Check sheet for the modelled part. Datum: model origin and axes. Units: mm. Face numbers are marked on the shaded views. A direction names the side the tool comes from. Round coordinates to 2 decimals unless told otherwise and drop trailing zeros. Loops run counter-clockwise (first coordinate to the right, second up) from the corner with the lowest first, then second, coordinate; pieces in that order, holes last. Notation, with made-up numbers: M 52.5,68.25 L 102.5,68.25 A19 cw 102.5,81.25 Z; hole C 78.5,59.25 d6. An arc over 180 degrees is marked long. One line per question, with ' | ' between items. Start each with the question number.
(1) Draft check along X on the marked faces 3, 4 and 5. Enter one of: +X half, -X half, draft (parallel to the pull), parting line (faces both ways), or undercut.
(2) Thickness scan on probe 1 along Z at (x, y) = (-44, -1); probe 2 along X at (y, z) = (-3.5, 36); probe 3 along Y at (x, z) = (-59, 32) (3 decimals). Record the ranges inside material, lowest first. Write a range as [from, to].
(3) Section check B-B (y = -4.25). Record the boundary of the cut face in (x, z) (3 decimals).
(4) Go/stop test with flat-tipped pins: P1, Ø2, axis at y = -2.5, z = 44.5, coming from the -X side; P2, Ø1, axis at x = -41.5, y = -4.5, coming from the -Z side; P3, Ø1.5, axis at y = -4.5, z = 38, coming from the +X side. Record where each tip stops, or that it passes through.
(5) Tool access check on the marked faces 1 and 2. Record the directions out of +Z, -Z, +X, -X, +Y, -Y that give a thin tool (end or side, any length) a straight path to the whole face; none if there is none.
(6) Section check A-A (y = 0.75). Record the boundary of the cut face in (x, z), and give its area (3 significant figures).
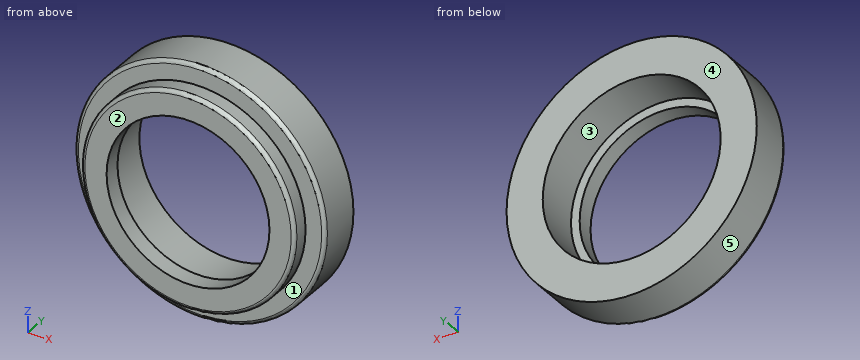
```python
from build123d import *

# Parameters (mm, degrees)
F0_R     = 17.89
F0_R_2   = 12.72
F1_DEPTH = 3.135
F3_R     = 15.25
F3_R_2   = 11.645
F4_DEPTH = 2.41
F5_R     = 0.5


with BuildPart() as f1:
    # F0 (on Front) → F1 (new body, symmetric)
    with BuildSketch(Plane.XZ):
        with Locations((-42.8615688275, 33.3970142528)):
            Circle(F0_R)
        with Locations((-42.8615688275, 33.3970142528)):
            Circle(F0_R_2, mode=Mode.SUBTRACT)
    extrude(amount=F1_DEPTH, both=True)

    # F3 (on offset) → F4 (join)
    with BuildSketch(Plane.XZ.offset(3.135)):
        with Locations((-43.0275388062, 33.2303009927)):
            Circle(F3_R)
        with Locations((-43.0275388062, 33.2303009927)):
            Circle(F3_R_2, mode=Mode.SUBTRACT)
    extrude(amount=F4_DEPTH)

    # F5
    f5_edges = [f1.edges().sort_by_distance(p)[0] for p in [
        (-58.277539, -5.545, 33.230301),
        (-60.751569, -3.135, 33.397014),
    ]]
    fillet(f5_edges, radius=F5_R)


solid = f1.part
```
The answers:
1) face 3: undercut | face 4: draft | face 5: parting line
2) probe 1: [15.54, 20.73], [46.07, 51.25] | probe 2: [-58.02, -54.34], [-31.72, -28.03] | probe 3: [-3.135, 3.135]
3) outline: C -43.028,33.23 d30.5; hole C -43.028,33.23 d23.29
4) P1: x = -57.63 | P2: z = 18.01 | P3: x = -28.32
5) face 1: -Y | face 2: +Z, -Z, +X, -X, -Y
6) outline: C -42.86,33.4 d35.78; hole C -42.86,33.4 d25.44 | area: 497 mm²
